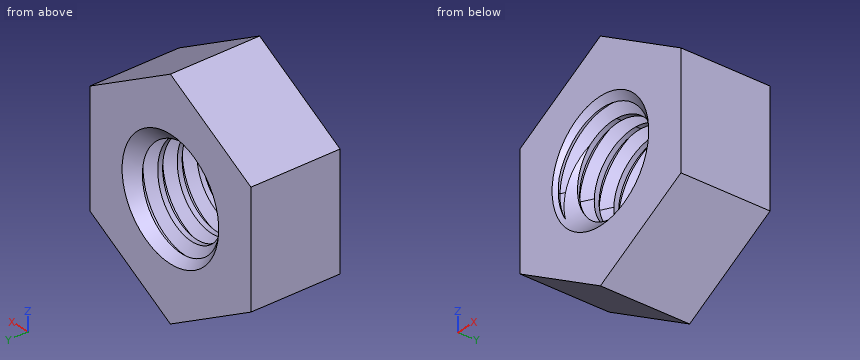
```python
from build123d import *

# Parameters (mm, degrees)
BOSS_EXTRUDE1_DEPTH = 3.2
SKETCH2_R           = 1.6
CUT_EXTRUDE1_DEPTH  = 3.2
CHAMFER1_SIZE       = 0.5
THREAD1_PITCH       = 0.7


with BuildPart() as part:
    # Sketch1 → Boss-Extrude1 (new body)
    with BuildSketch(Plane(origin=(0, 0, 0), x_dir=(1, 0, 0), z_dir=(0, 1, 0))):
        Polygon((0, 4.041451884), (-3.5, 2.020725942), (-3.5, -2.020725942), (0, -4.041451884), (3.5, -2.020725942), (3.5, 2.020725942), align=None)
    extrude(amount=BOSS_EXTRUDE1_DEPTH)

    # Sketch2 → Cut-Extrude1 (cut)
    with BuildSketch(Plane(origin=(0, 3.2, 0), x_dir=(1, 0, 0), z_dir=(0, 1, 0))):
        with Locations(Location((0, 0, 0), (0, 0, 270))):
            Circle(SKETCH2_R)
    extrude(amount=-CUT_EXTRUDE1_DEPTH, mode=Mode.SUBTRACT)

    # Chamfer1
    chamfer1_edges = [part.edges().sort_by_distance(p)[0] for p in [
        (0, 0, -1.6),
        (0, 3.2, -1.6),
    ]]
    chamfer(chamfer1_edges, length=CHAMFER1_SIZE)

    # Thread1: the profile of Thread Profile1 profile screwed along a right-hand helix of 4.571429 turns, 6 arcs to a turn; built about Z, then put on its axis
    thread1_z = Axis((0, 0, 0), (0, 0, 1))
    thread1_corners = [(1.5997, 0, -0.000173205), (1.978886113, -1e-09, 0.218749999), (1.978886113, -1e-09, 0.306249999), (1.5997, 0, 0.525173203)]
    with BuildLine(mode=Mode.PRIVATE) as thread1_profile:
        Line(thread1_corners[0], thread1_corners[1])
        Line(thread1_corners[1], thread1_corners[2])
        Line(thread1_corners[2], thread1_corners[3])
        Line(thread1_corners[3], thread1_corners[0])
    thread1_cap = Face(thread1_profile.wire())
    thread1_turn_angles = [0, 30, 60, 90, 120, 150, 180, 210, 240, 270, 300, 330, 360]
    thread1_turn_weights = [1, 0.8660254037844387, 1, 0.8660254037844387, 1, 0.8660254037844387, 1, 0.8660254037844387, 1, 0.8660254037844387, 1, 0.8660254037844387, 1]
    thread1_turn_rails = [Edge.make_bspline([Vector(p[0], p[1], 0).rotate(thread1_z, thread1_turn_angles[k]) / thread1_turn_weights[k] + Vector(0, 0, p[2] + THREAD1_PITCH * thread1_turn_angles[k] / 360) for k in range(13)], [0, 0, 0, 1, 1, 2, 2, 3, 3, 4, 4, 5, 5, 6, 6, 6], 2, thread1_turn_weights) for p in thread1_corners]
    thread1_turn_sides = [Face.make_surface_from_curves(thread1_turn_rails[p[0]], thread1_turn_rails[p[1]]) for p in [(0, 1), (1, 2), (2, 3), (3, 0)]]
    thread1_last_angles = [1440, 1470, 1500, 1530, 1560, 1590, 1620, 1632.857142857, 1645.714285714]
    thread1_last_weights = [1, 0.8660254037844387, 1, 0.8660254037844387, 1, 0.8660254037844387, 1, 0.9749279121818266, 1]
    thread1_last_rails = [Edge.make_bspline([Vector(p[0], p[1], 0).rotate(thread1_z, thread1_last_angles[k]) / thread1_last_weights[k] + Vector(0, 0, p[2] + THREAD1_PITCH * thread1_last_angles[k] / 360) for k in range(9)], [0, 0, 0, 1, 1, 2, 2, 3, 3, 4, 4, 4], 2, thread1_last_weights) for p in thread1_corners]
    thread1_last_sides = [Face.make_surface_from_curves(thread1_last_rails[p[0]], thread1_last_rails[p[1]]) for p in [(0, 1), (1, 2), (2, 3), (3, 0)]]
    thread1 = Plane(origin=(0, 3.2, 0), x_dir=(-0.999390827, 0, -0.034899497), z_dir=(0, -1, 0)) * Solid(Shell([*[p.moved(Location((0, 0, THREAD1_PITCH * i))) for i in range(4) for p in thread1_turn_sides], *thread1_last_sides, thread1_cap, thread1_cap.rotate(thread1_z, 1645.714285714).moved(Location((0, 0, THREAD1_PITCH * 1645.714285714 / 360)))]))
    add(thread1, mode=Mode.SUBTRACT)


solid = part.part
```
Verification items for the finished model (mm, model axes). Coordinates: 2 decimals unless noted, no trailing zeros. Write each loop counter-clockwise with the first axis right and the second up, starting at its lowest first coordinate (ties: lowest second). Pieces come first, ordered by that corner, then holes. Notation, with made-up numbers: (19.25, 42) - (78.25, 42) arc R14 cw to (78.25, 63) - close; hole circle Ø4 at (49.25, 37.25). An arc over 180 degrees is marked (long way). Write item = value, one per line.
Q1. Material ranges on L1, parallel to X at y = 1.9, z = 0; L2, parallel to X at y = 3.05, z = -0.5; L3, parallel to Z at x = 1, y = 0.2, recorded low to high. Write a range as from..to.
Answer:
L1 = -3.5..-1.6, 1.98..3.5
L2 = -3.5..-1.88, 1.88..3.5
L3 = -3.46..-1.62, 1.62..3.46
Q2. Cross-section at B-B (x = 2.25). Enter the section's corners in (y, z).
Answer:
outline = (0, -2.74) - (3.2, -2.74) - (3.2, 2.74) - (0, 2.74) - close
Q3. Cross-section at A-A (z = -2.75). Enter the section's corners in (x, y), plus the area to 3 significant figures.
Answer:
outline = (-2.24, 0) - (2.24, 0) - (2.24, 3.2) - (-2.24, 3.2) - close
area = 14.3 mm²
Q4. Go/stop test with a flat-tipped pin: pin 1 Ø1.5 at (x, z) = (2.5, -2.5) entering from -Y. Record where the tip stops, or that it passes through.
Answer:
pin_1 = 0
